from build123d import *

# Parameters (mm, degrees)
BOSS_EXTRUDE1_DEPTH = 20
CUT_EXTRUDE1_REACH  = 22
SKETCH2_R           = 2.55
CUT_EXTRUDE2_REACH  = 22
SKETCH3_R           = 2.55


with BuildPart() as part:
    # Sketch1 → Boss-Extrude1 (new body)
    with BuildSketch(Plane.XY):
        Polygon((0, 20), (0, 0), (20, 0), (20, 3), (3, 3), (3, 20), align=None)
    extrude(amount=BOSS_EXTRUDE1_DEPTH)

    # Sketch2 → Cut-Extrude1 (cut, up to next)
    with BuildSketch(Plane.ZY, mode=Mode.PRIVATE) as cut_extrude1_sk1:
        with Locations((10, 10)):
            Circle(SKETCH2_R)
    cut_extrude1_tool1 = extrude(cut_extrude1_sk1.sketch, amount=-CUT_EXTRUDE1_REACH, mode=Mode.PRIVATE) & part.part
    add(cut_extrude1_tool1.solids().sort_by_distance((0, 10, 10))[0], mode=Mode.SUBTRACT)

    # Sketch3 → Cut-Extrude2 (cut, up to next)
    with BuildSketch(Plane.XZ, mode=Mode.PRIVATE) as cut_extrude2_sk1:
        with Locations((10, 10)):
            Circle(SKETCH3_R)
    cut_extrude2_tool1 = extrude(cut_extrude2_sk1.sketch, amount=-CUT_EXTRUDE2_REACH, mode=Mode.PRIVATE) & part.part
    add(cut_extrude2_tool1.solids().sort_by_distance((10, 0, 10))[0], mode=Mode.SUBTRACT)


solid = part.part
CAD build for the part. Positions are in the model's coordinates, mm. A direction names the side the tool comes from. Give positions to 0.01 mm unless a question says otherwise; leave off trailing zeros. Order: outer loops, then holes, each group sorted by start corner. A loop starts at its lowest first (then second) coordinate and runs counter-clockwise, first axis right, second up. Notation, with made-up numbers: (-3.75, 44.5) - (1.25, 44.5) arc R29 cw to (1.25, 78.5) - close; hole circle Ø11 at (42.5, 17.5). An arc over 180 degrees is marked (long way). Write each question's results on one line, items separated by ' | '.
1. Saw through at C-C on x = 10. List the corners of the cut face in (y, z).
Calculated:
outline: (0, 0) - (3, 0) - (3, 7.45) - (0, 7.45) - close; (0, 12.55) - (3, 12.55) - (3, 20) - (0, 20) - close
2. Probe L1, parallel to Z at x = 10, y = 2.35; L2, parallel to Y at x = 4.75, z = 14. List the from-to ranges inside material, lowest first. Write a range as from..to.
Calculated:
L1: z = 0..7.45, 12.55..20 | L2: y = 0..3
3. Pin check, flat tips, straight feed: pin 1 (12 mm diameter, centred on y = 17.5, z = 14, fed in from +X); pin 2 (1 mm diameter, centred on x = 13, z = 12, fed in from +Y). Stop position of each tip, or through.
Calculated:
pin 1: stops at x = 3 | pin 2: stops at y = 3
4. Saw through at B-B on z = 10. List the corners of the cut face in (x, y), and give its area (3 significant figures).
Calculated:
outline: (0, 0) - (7.45, 0) - (7.45, 3) - (3, 3) - (3, 7.45) - (0, 7.45) - close; (0, 12.55) - (3, 12.55) - (3, 20) - (0, 20) - close; (12.55, 0) - (20, 0) - (20, 3) - (12.55, 3) - close | area: 80.4 mm2
5. Saw through at D-D on z = 7.75. List the corners of the cut face in (x, y).
Calculated:
outline: (0, 0) - (8.8, 0) - (8.8, 3) - (3, 3) - (3, 8.8) - (0, 8.8) - close; (0, 11.2) - (3, 11.2) - (3, 20) - (0, 20) - close; (11.2, 0) - (20, 0) - (20, 3) - (11.2, 3) - close
6. 3-axis set-ups, long thin cutter, end or side, ignore diameter. For faces 1 (the face through (2, 20, 10)), 2 (the face through (3, 13, 10)): which of +Z, -Z, +X, -X, +Y, -Y reach the whole face in a straight line?
Calculated:
face 1: +Z, -Z, +X, -X, +Y | face 2: +Z, -Z, +X, +Y
7. Pull direction Y, two halves, no side cores. Call faces 3 (the face through (1.48, 7.74, 11.18)), 4 (the face through (11.18, 1.48, 7.74)), 5 (the face through (14, 3, 10)): released by +Y, released by -Y, zero draft, split by the parting line, or undercut.
Calculated:
face 3: undercut | face 4: zero draft | face 5: released by +Y
8. Saw through at A-A on y = 7.75. List the corners of the cut face in (x, z).
Calculated:
outline: (0, 0) - (3, 0) - (3, 8.8) - (0, 8.8) - close; (0, 11.2) - (3, 11.2) - (3, 20) - (0, 20) - close
